The drawing under review shows one solid part. Ordinate dimensions are in mm from its lowest x, y, z. Coordinates: 2 decimals unless noted, no trailing zeros. Loops run counter-clockwise (first coordinate to the right, second up) from the corner with the lowest first, then second, coordinate; pieces in that order, holes last.
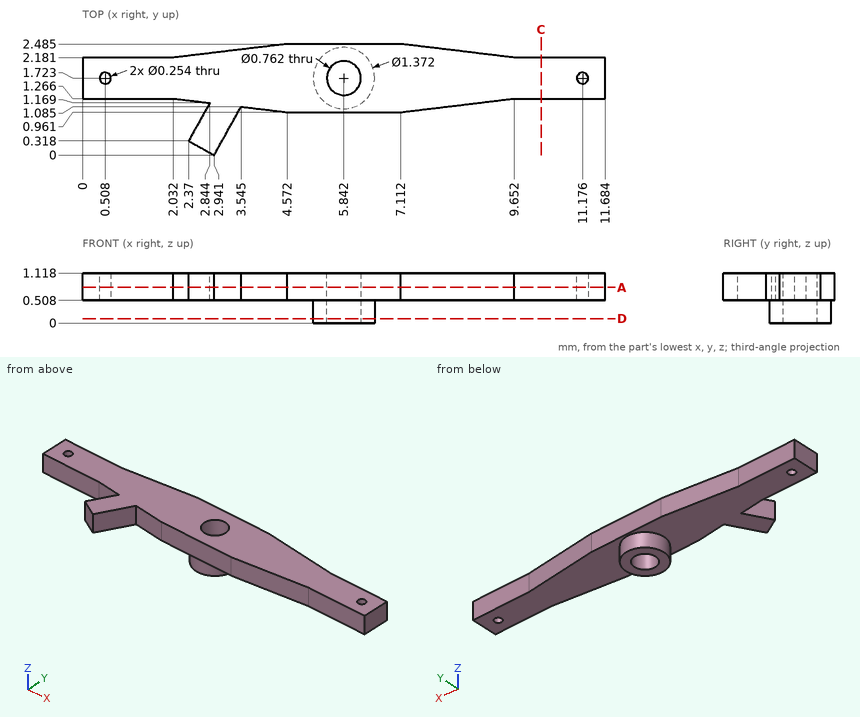
Q1. Take a section at C-C, the plane x = 10.25. Write out the cut boundary in (y, z).
Q2. Take a section at D-D, the plane z = 0.1. Write out the cut boundary in (x, y) (1 decimal).
Q3. For line 1 (X direction, y = 1.7, z = 0.45); line 2 (Z direction, x = 11, y = 1.5); line 3 (Y direction, x = 4.75, z = 0.6) (1 decimal), list the stretches that pass through material, from the lowest coordinate up.
Q4. Take a section at A-A, the plane z = 0.8. Write out the cut boundary in (x, y) (1 decimal).
Q5. Clearance check with a flat-ended pin moving along its axis: pin 1 Ø0.5 at (x, z) = (1, 0.5) entering from -Y. State where the tip first meets the part, or that it passes through.
Entries:
1. outline: (1.27, 0.51) - (2.18, 0.51) - (2.18, 1.12) - (1.27, 1.12) - close
2. outline: circle Ø1.4 at (5.8, 1.7); hole circle Ø0.8 at (5.8, 1.7)
3. line 1: x = 5.16 to 5.46, 6.22 to 6.53
3. line 2: z = 0.51 to 1.12
3. line 3: y = 1 to 2.5
4. outline: (0, 1.3) - (2, 1.3) - (2.8, 1.2) - (2.4, 0.3) - (2.9, 0) - (3.5, 1.1) - (4.6, 1) - (7.1, 1) - (9.7, 1.3) - (11.7, 1.3) - (11.7, 2.2) - (9.7, 2.2) - (7.1, 2.5) - (4.6, 2.5) - (2, 2.2) - (0, 2.2) - close; hole circle Ø0.3 at (0.5, 1.7); hole circle Ø0.8 at (5.8, 1.7); hole circle Ø0.3 at (11.2, 1.7)
5. pin 1: stops at y = 1.27
